For this review, take the finished solid that the model builds, in its own axes (mm). A direction names the side the tool comes from. Round coordinates to 2 decimals unless told otherwise and drop trailing zeros. Order: outer loops, then holes, each group sorted by start corner. A loop starts at its lowest first (then second) coordinate and runs counter-clockwise, first axis right, second up. Notation, with made-up numbers: (39, -25.75) - (67, -25.75) arc R26 cw to (67, 7.25) - close; hole circle Ø9 at (65.25, 85.25). An arc over 180 degrees is marked (long way). Write each question's results on one line, items separated by ' | '. Start each with the question number.
(1) For faces 1 (the flat face through (471, 1, -4)), 2 (the flat face through (234, 1.5, -8)), list the 3-axis set-ups (+Z, -Z, +X, -X, +Y, -Y) from which the entire face can be reached by the end or side of a thin tool; tool diameter is ignored.
(2) Insertion check: pin 1 Ø5 at (x, y) = (426, 10) entering from -Z; pin 2 Ø3 at (x, z) = (423.5, -4.5) entering from +Y. Each pin has a flat end and moves straight along its axis. Give the tip position at first contact, or say it passes through.
(3) For L1, parallel to Z at x = 45, y = 7.75; L2, parallel to Y at x = 266, z = -2.25; L3, parallel to X at y = 0.5, z = -11.75, list the stretches that pass through material, from the lowest coordinate up. Write a range as from..to.
(4) Take a section at B-B, the plane z = -4.5. Give the boundary of the cut face in (x, y).
(5) Take a section at C-C, the plane y = 12. Give the boundary of the cut face in (x, z), plus the area to 3 significant figures.
(6) Take a section at A-A, the plane x = 70. Give the boundary of the cut face in (y, z).
```python
from build123d import *

# Parameters (mm, degrees)
EXTRUDE_1_DEPTH     = 475
CUT_EXTRUDE_1_DEPTH = 16


with BuildPart() as part:
    # Эскиз1 → Бобышка-Вытянуть1 (new body)
    with BuildSketch(Plane(origin=(0, 0, 0), x_dir=(0, 0, -1), z_dir=(1, 0, 0))):
        Polygon((0, 0), (0, 15), (1.5, 15), (1.5, 1.5), (15, 1.5), (15, 0), align=None)
    extrude(amount=EXTRUDE_1_DEPTH)

    # Эскиз2 → Вырез-Вытянуть1 (cut, through all)
    with BuildSketch(Plane.XZ):
        Polygon((475, 0), (454.951956964, -20.048043036), (475, -20.048043036), align=None)
    cut_extrude_1 = extrude(amount=-CUT_EXTRUDE_1_DEPTH, mode=Mode.SUBTRACT)

    # Зеркальное отражение1: Вырез-Вытянуть1 across plane
    add(cut_extrude_1.mirror(Plane(origin=(237.5, 0, 0), x_dir=(0, 0, 1), z_dir=(1, 0, 0))), mode=Mode.SUBTRACT)


solid = part.part
```
Results below:
1) face 1: -Z, +X, +Y, -Y | face 2: -Z, +X, -X, +Y
2) pin 1: stops at z = -1.5 | pin 2: stops at y = 1.5
3) L1: z = -1.5..0 | L2: y = 0..1.5 | L3: x = 11.75..463.25
4) outline: (4.5, 0) - (470.5, 0) - (470.5, 1.5) - (4.5, 1.5) - close
5) outline: (0, 0) - (1.5, -1.5) - (473.5, -1.5) - (475, 0) - close | area: 710 mm^2
6) outline: (0, -15) - (1.5, -15) - (1.5, -1.5) - (15, -1.5) - (15, 0) - (0, 0) - close
